Source: CAD feature listing. Evaluate the final solid. Frame: model axes, mm. A direction names the side the tool comes from. Give positions to 0.01 mm unless a question says otherwise; leave off trailing zeros. Loops run counter-clockwise (first coordinate to the right, second up) from the corner with the lowest first, then second, coordinate; pieces in that order, holes last.
Autodesk Inventor part; units mm, degrees
ref_plane "YZ Plane" through (0, 0, 0) normal (1, 0, 0) x (0, 1, 0)
ref_plane "XZ Plane" through (0, 0, 0) normal (0, 1, 0) x (-1, 0, 0)
ref_plane "XY Plane" through (0, 0, 0) normal (0, 0, 1) x (1, 0, 0)
sketch "スケッチ1" plane through (0, 0, 0) normal (0, 1, 0) x (-1, 0, 0)
  circle A0 centre (0, 0) radius 2
  circle A1 centre (0, 0) radius 1.15
  line L0 (0, 0) -> (2, 0)
  line L1 (2, 0) -> (2, -5)
  line L2 (2, -5) -> (0, -5)
  line L3 (0, -5) -> (0, 0)
  line L4 (0, 0) -> (2, 0)
  line L5 (2, 0) -> (2, 4)
  line L6 (2, 4) -> (0, 4)
  line L7 (0, 4) -> (0, 0)
  circle A2 centre (0, 0) radius 3
  circle A3 centre (0, 0) radius 2.5
  line L8 (0, 0) -> (2.5, 0)
  line L9 (2.5, 0) -> (2.5, 2.6782)
  line L10 (2.5, 2.6782) -> (0, 2.6782)
  line L11 (0, 2.6782) -> (0, 0)
  line L12 (0, 2.6782) -> (7, 2.6782)
  line L13 (7, 2.6782) -> (7, -5)
  line L14 (7, -5) -> (0, -5)
  line L15 (0, -5) -> (0, 2.6782)
  point P0 (0, 2)
  point P1 (0, -2)
  dimension "d0" = 4
  dimension "d1" = 2.3
  dimension "d2" = 5
  dimension "d3" = 4
  dimension "d4" = 6
  dimension "d6" = 5
  dimension "d7" = 2.5
  dimension "d8" = 7
sketch "スケッチ2" plane through (0, 0, 0) normal (0, 1, 0) x (-1, 0, 0)
  line L0 (0, -1.1495) -> (-5, -1.1495)
  line L1 (-5, -1.1495) -> (-5, -1.9793)
  line L2 (-5, -1.9793) -> (0, -1.9793)
  line L3 (0, -1.9793) -> (0, -1.1495)
  line L4 (-5, -1.9793) -> (-6.828, -1.9793)
  line L5 (-6.828, -1.9793) -> (-6.828, 0)
  line L6 (-6.828, 0) -> (-5, 0)
  line L7 (-5, 0) -> (-5, -1.9793)
  line L8 (0, 1.115) -> (-6.6551, 1.115)
  line L9 (-6.6551, 1.115) -> (-6.6551, 1.9793)
  line L10 (-6.6551, 1.9793) -> (0, 1.9793)
  line L11 (0, 1.9793) -> (0, 1.115)
  point P0 (0, 0)
  dimension "d5" = 5
extrude "押し出し1" add sketch "スケッチ1" along normal blind 4.6 contours L8 A3 L1 | A0 L7 A3 L5 | L5 A3 L8 | A3 L9 A2 L1 | A3 L7 L10 A2 L5 | L5 A2 L9 A3 | A2 L9 L12 L13 L14 L1 | A2 L10 L5 | L5 L10 L9 A2
extrude "押し出し2" add sketch "スケッチ1" against normal blind 1 contours L0 A1 L7 A0 | L1 A3 L3 A0 | A0 L3 A1 L0 | L8 A3 L1 | A0 L7 A3 L5 | L5 A3 L8 | L7 A1 L3 A0 | A3 L9 A2 L1 | L1 A2 L3 A3 | A3 L7 L10 A2 L5 | L5 A2 L9 A3 | A2 L9 L12 L13 L14 L1 | L1 L2 L3 A2 | A2 L10 L5 | L5 L10 L9 A2
sketch "スケッチ3" plane through (0, 4.6, 0) normal (0, 1, 0) x (1, 0, 0)
  circle A0 centre (0, 0) radius 1.15
  line L0 (-2, 0) -> (-2, 5)
  circle A1 centre (0, 0) radius 2
  line L1 (0, -2) -> (0, -2.6782)
  line L2 (-7, 5) -> (0, 5)
  line L3 (0, -2.6782) -> (-7, -2.6782)
  line L4 (-7, -2.6782) -> (-7, 5)
  line L5 (-7, 5) -> (0, 5)
  line L6 (0, 5) -> (0, -2.6782)
  point P0 (0, 2)
extrude "押し出し3" add sketch "スケッチ3" along normal blind 1 contours A0 L6 A1 | A0 L6 A1 | A1 L0 L2 L6 | L1 L3 L4 L2 L0 A1
sketch "スケッチ4" plane through (-7, -1, 2.6782) normal (0, 0, 1) x (1, 0, 0)
  line L0 (7, 6.6) -> (0, 6.6)
  line L1 (0, 6.6) -> (2.5, 6.6)
  line L2 (2.5, 6.6) -> (2.5, 3.35)
  line L3 (2.5, 3.35) -> (0, 3.35)
  line L4 (0, 3.35) -> (0, 6.6)
  circle A0 centre (2.5, 3.35) radius 1.55
  line L5 (5, 1) -> (7, 1)
  line L6 (7, 1) -> (5.5, 1)
  line L7 (5.5, 1) -> (5.5, 1.5)
  line L8 (5.5, 1.5) -> (7, 1.5)
  line L9 (7, 1.5) -> (7, 1)
  circle A1 centre (5.5, 1.5) radius 0.5
  dimension "d15" = 2.5
  dimension "d16" = 3.25
  dimension "d17" = 3.1
  dimension "d18" = 1.5
  dimension "d19" = 0.5
extrude "押し出し4" cut sketch "スケッチ4" against normal blind 6 contours A0 L3 L2 | L2 L3 A0 | A1 L8 L7 | L7 L8 A1
properties part number "rod5.0"
1) Cut plane D-D (x = -4.5). Return loops of the section in (y, z), and give its area (3 significant figures).
Checks:
outline: (-1, -5) - (5.6, -5) - (5.6, 2.68) - (3.9, 2.68) - (3.9, -3.32) - (0.8, -3.32) - (0.8, 2.68) - (-1, 2.68) - close
area: 32.1 mm2
2) Contact query for flat-ended pins moving along their axis: P1, Ø3.5, axis at y = 2.5, z = -1.5, coming from the +X side; P2, Ø0.5, axis at y = 5, z = -3.5, coming from the +X side; P3, Ø3, axis at y = 2, z = -1, coming from the +X side. Output: stop coordinate, or through.
Checks:
P1: stops at x = -1.98
P2: stops at x = 0
P3: stops at x = -1.94
3) Cut plane C-C (y = 2.35). Return loops of the section in (x, z), and give its area (3 significant figures).
Checks:
outline: (-7, -5) - (-2, -5) - (-2, 0) arc R2 cw to (0, 2) - (0, 2.68) - (-2.95, 2.68) - (-2.95, -3.32) - (-6.05, -3.32) - (-6.05, 2.68) - (-7, 2.68) - close
area: 22.0 mm2
4) Ray query, probe 1 along Y at (x, z) = (-4.5, -0.4); probe 2 along Y at (x, z) = (1.5, 1); probe 3 along X at (y, z) = (-0.5, -3). Return the intervals inside material, ascending.
Checks:
probe 1: y = -1 to 0.8, 3.9 to 5.6
probe 2: y = -1 to 0, 4.6 to 5.6
probe 3: x = -7 to 0
5) Pull-direction query (Y, two-part tool) for faces 1 (the flat face through (0, 5, -4)), 2 (the cylindrical face through (-1.4, 2.78, 1.43)), 3 (the flat face through (-3, -1, -1)); classes: released by +Y, released by -Y, zero draft, split by the parting line, or undercut.
Checks:
face 1: zero draft
face 2: undercut
face 3: released by -Y
6) Cut plane B-B (z = -2.25). Return loops of the section in (x, y), and give its area (3 significant figures).
Checks:
outline: (-7, -1) - (0, -1) - (0, 0) - (-2, 0) - (-2, 4.6) - (0, 4.6) - (0, 5.6) - (-7, 5.6) - close; hole circle Ø3.1 at (-4.5, 2.35)
area: 29.5 mm2
7) Cut plane A-A (y = 5). Return loops of the section in (x, z).
Checks:
outline: (-7, -5) - (0, -5) - (0, -2) arc R2 ccw to (0, 2) - (0, 2.68) - (-7, 2.68) - close; hole circle Ø2.3 at (0, 0)
8) Reachability of faces 4 (the flat face through (0, -0.5, -3.5)), 5 (the flat face through (-2, 2, -2)), 6 (the flat face through (-5, 2, -3.322)), 7 (the cylindrical face through (2, 5, 0)), 8 (the cylindrical face through (-2, 0.5, 2)) from +Z, -Z, +X, -X, +Y, -Y: full face, straight path, thin tool, end or side. Return the list, or none.
Checks:
face 4: -Z, +X, +Y, -Y
face 5: -Z, +X
face 6: +Z
face 7: +X, +Y, -Y
face 8: +Z, -Z
